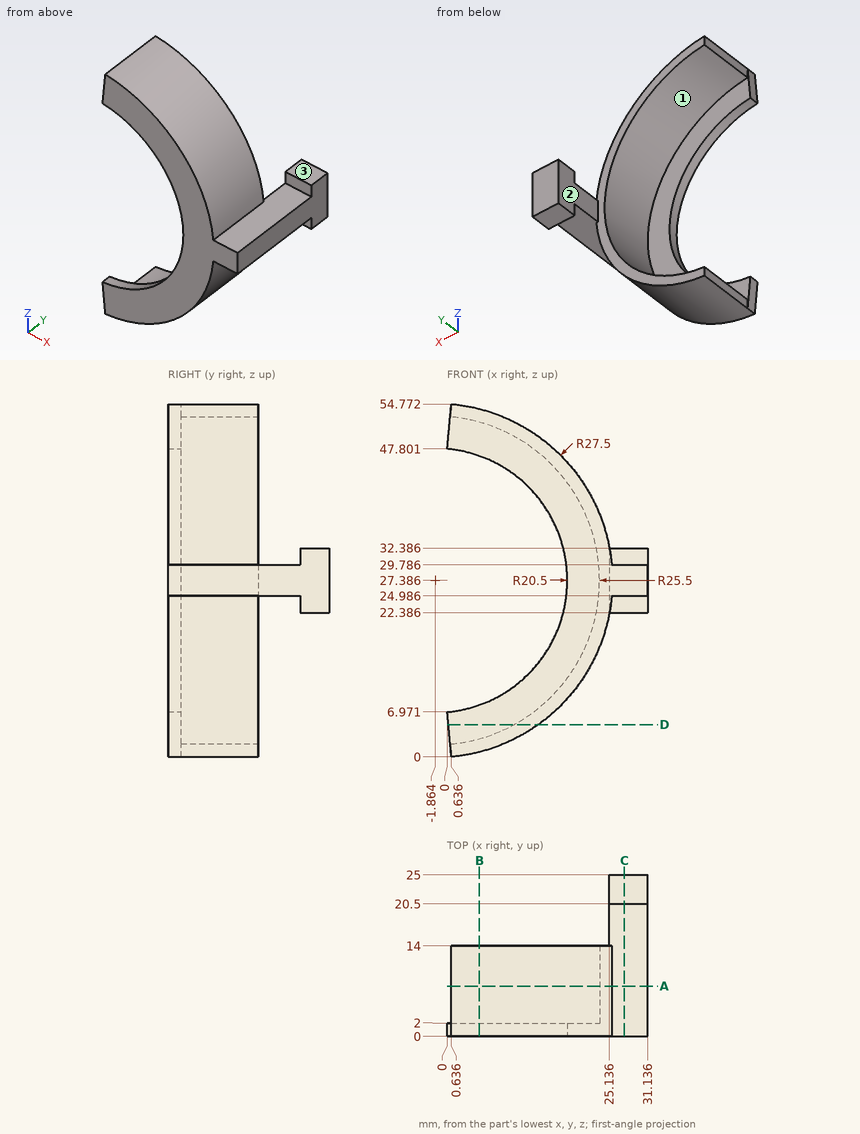
Answer from the drawing. Dimensions are ordinates in mm from the lowest x, y and z of the part. A direction names the side the tool comes from. Round coordinates to 2 decimals unless told otherwise and drop trailing zeros. Write each loop counter-clockwise with the first axis right and the second up, starting at its lowest first coordinate (ties: lowest second). Pieces come first, ordered by that corner, then holes. Notation, with made-up numbers: (-15, -30) - (9, -30) arc R29 ccw to (9, -10) - close; hole circle Ø5 at (85, -19). An arc over 180 degrees is marked (long way). Use a Markdown table: item, result.
(1) The part is cut by section C-C (x = 27.5). Write down the section's boundary in (y, z).
Reported:
| item | result |
|---|---|
| outline | (0, 24.99) - (20.5, 24.99) - (20.5, 22.39) - (25, 22.39) - (25, 32.39) - (20.5, 32.39) - (20.5, 29.79) - (0, 29.79) - close |
(2) Which of the six approach directions +Z, -Z, +X, -X, +Y, -Y give full straight-line access (tool end or side, diameter ignored) to the marked faces 1, 2 and 3?
Reported:
| item | result |
|---|---|
| face 1 | -X, +Y |
| face 2 | +Z, -Z, -X, +Y |
| face 3 | +Z, +X, -X, +Y, -Y |
(3) The part is cut by section A-A (y = 7.75). Write down the section's boundary in (x, z), then the cut area to 3 significant figures.
Reported:
| item | result |
|---|---|
| outline | (0.64, 0) arc R27.5 ccw to (25.53, 24.99) - (31.14, 24.99) - (31.14, 29.79) - (25.53, 29.79) arc R27.5 ccw to (0.64, 54.77) - (0.64, 52.76) arc R25.5 cw to (0.64, 2.01) - close |
| area | 183 mm2 |
(4) Straight lines are drawn through the part: line 1 along Y through (x, z) = (17.5, 35); line 2 along Z through (x, y) = (26.5, 6.25); line 3 along X through (y, z) = (23.25, 27). For each, find the intervals that lie inside material, in ascending order. Write a range as [from, to].
Reported:
| item | result |
|---|---|
| line 1 | [0, 2] |
| line 2 | [24.99, 29.79] |
| line 3 | [25.14, 31.14] |
(5) The part is cut by section D-D (z = 5). Write down the section's boundary in (x, y).
Reported:
| item | result |
|---|---|
| outline | (0.18, 0) - (14.11, 0) - (14.11, 14) - (10.35, 14) - (10.35, 2) - (0.18, 2) - close |
(6) Each of these flat-tipped pins is pushed along its axis until it touches: pin 1 Ø2 at (y, z) = (14.5, 25.5) entering from -X; pin 2 Ø6.5 at (x, y) = (26.5, 7.5) entering from +Z; pin 3 Ø1 at (y, z) = (10.5, 54) entering from -X; pin 4 Ø12 at (y, z) = (18.5, 17.5) entering from +X. Where does it stop, or does it pass through?
Reported:
| item | result |
|---|---|
| pin 1 | x = 23.49 |
| pin 2 | z = 38.59 |
| pin 3 | x = 0.64 |
| pin 4 | x = 31.14 |
(7) The part is cut by section B-B (x = 5). Write down the section's boundary in (y, z) (1 decimal).
Reported:
| item | result |
|---|---|
| outline | (0, 0.8) - (14, 0.8) - (14, 2.8) - (2, 2.8) - (2, 8.1) - (0, 8.1) - close; (0, 46.7) - (2, 46.7) - (2, 51.9) - (14, 51.9) - (14, 54) - (0, 54) - close |
